Here's how the part is built. I have some questions about the finished solid (model axes, mm). Face numbers are marked on the shaded views. Give positions to 0.01 mm unless a question says otherwise; leave off trailing zeros. Order: outer loops, then holes, each group sorted by start corner. A loop starts at its lowest first (then second) coordinate and runs counter-clockwise, first axis right, second up. Notation, with made-up numbers: M 25.5,-27 L 32.5,-27 A16 cw 32.5,-20 Z; hole C -14.75,-24 d8. An arc over 180 degrees is marked long. Use CSV: the item, a comma, the result in double quotes. Start each with the question number.
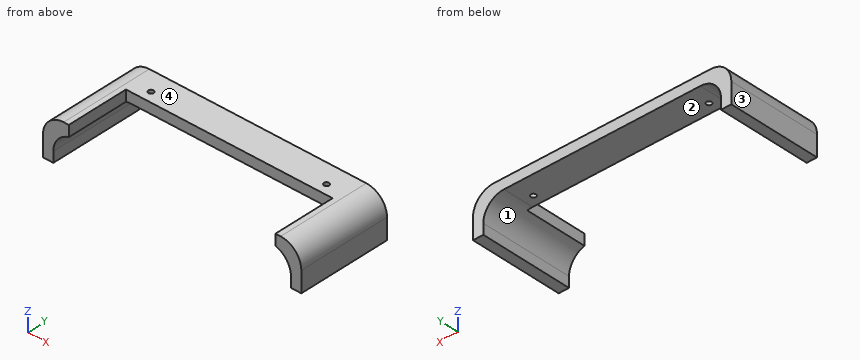
```python
from build123d import *

# Parameters (mm, degrees)
SKETCH1_W               = 250
SKETCH1_H               = 250
SKETCH1_W_2             = 230
SKETCH1_H_2             = 230
BOSS_EXTRUDE1_DEPTH     = 90
SKETCH2_W               = 200
SKETCH2_H               = 60
CUT_EXTRUDE1_DEPTH      = 50
FILLET1_R               = 20
SKETCH10_W              = 210
SKETCH10_H              = 90
CUT_EXTRUDE6_DEPTH      = 1
CUT_EXTRUDE6_DEPTH_BACK = 251
SKETCH11_R              = 2.5
CUT_EXTRUDE7_DEPTH      = 10


with BuildPart() as part:
    # Sketch1 → Boss-Extrude1 (new body)
    with BuildSketch(Plane(origin=(0, 0, 0), x_dir=(1, 0, 0), z_dir=(0, 1, 0))):
        Rectangle(SKETCH1_W, SKETCH1_H)
        Rectangle(SKETCH1_W_2, SKETCH1_H_2, mode=Mode.SUBTRACT)
    extrude(amount=BOSS_EXTRUDE1_DEPTH)

    # Sketch2 → Cut-Extrude1 (cut)
    with BuildSketch(Plane.XY.offset(125)):
        with Locations((0, 30)):
            Rectangle(SKETCH2_W, SKETCH2_H)
    extrude(amount=-CUT_EXTRUDE1_DEPTH, mode=Mode.SUBTRACT)

    # Fillet1
    fillet1_edges = [part.edges().sort_by_distance(p)[0] for p in [
        (-115, 45, 115),
        (115, 45, 115),
        (115, 45, -115),
        (-115, 45, -115),
        (-125, 45, 125),
        (125, 45, 125),
        (125, 45, -125),
        (-125, 45, -125),
    ]]
    fillet(fillet1_edges, radius=FILLET1_R)

    # Sketch10 → Cut-Extrude6 (cut, two sides)
    with BuildSketch(Plane(origin=(125, 0, 0), x_dir=(0, 0, -1), z_dir=(1, 0, 0))) as cut_extrude6_sk:
        with Locations((20, 45)):
            Rectangle(SKETCH10_W, SKETCH10_H)
    extrude(amount=CUT_EXTRUDE6_DEPTH, mode=Mode.SUBTRACT)
    extrude(cut_extrude6_sk.sketch, amount=-CUT_EXTRUDE6_DEPTH_BACK, mode=Mode.SUBTRACT)

    # Sketch11 → Cut-Extrude7 (cut)
    with BuildSketch(Plane.XY.offset(125)):
        with Locations((-85, 70)):
            Circle(SKETCH11_R)
        with Locations((85, 70)):
            Circle(SKETCH11_R)
    extrude(amount=-CUT_EXTRUDE7_DEPTH, mode=Mode.SUBTRACT)


solid = part.part
```
Q1. Imagine slicing it at A-A, the plane x = 85. Please give me the cut outline in (y, z).
Q2. Imagine slicing it at B-B, the plane z = 122.5. Please give me the cut outline in (x, y).
Q3. I need wall thicknesses on line 1 (Y direction, x = 85, z = 117.75); line 2 (Y direction, x = -66, z = 118); line 3 (Z direction, x = -96, y = 71.5). Which ranges of each line are inside material? Lowest first, please. Write a range as [from, to].
Q4. For P1, Ø5.5, axis at x = -41.5, z = 120.5, coming from the -Y side; P2, Ø8.5, axis at y = 22.5, z = 117, coming from the -X side; P3, Ø3, axis at x = 85, y = 70, coming from the -Z side; P4, Ø24, axis at x = -2.5, y = 73.5, coming from the -Z side, each with a flat end and sliding along its axis, tell me the tip position at first contact or that it passes through.
Q5. We'd pull the mould along X, two halves only. Please class the marked faces 1, 2, 3 and 4: pulls with the +X half, pulls with the -X half, needs draft (parallel to the pull), parting line crosses it, or undercut.
Q6. Imagine slicing it at D-D, the plane x = -40. Please give me the cut outline in (y, z).
Q7. Imagine slicing it at C-C, the plane y = 80.5. Please give me the cut outline in (x, z).
Reply:
1,outline,"M 60,115 L 67.5,115 L 67.5,125 L 60,125 Z; M 72.5,115 L 90,115 L 90,125 L 72.5,125 Z"
2,outline,"M -114.68,0 L -100,0 L -100,60 L 100,60 L 100,0 L 114.68,0 L 114.68,90 L -114.68,90 Z; hole C -85,70 d5; hole C 85,70 d5"
3,line 1,"y = [60, 67.5], [72.5, 90]"
3,line 2,"y = [60, 90]"
3,line 3,"z = [114.97, 125]"
4,P1,"stops at y = 60"
4,P2,"stops at x = -123.44"
4,P3,"passes through"
4,P4,"stops at z = 115"
5,face 1,"undercut"
5,face 2,"undercut"
5,face 3,"pulls with the -X half"
5,face 4,"needs draft"
6,outline,"M 60,115 L 90,115 L 90,125 L 60,125 Z"
7,outline,"M -125,85 L -115,85 L -115,95 A20 cw -95,115 L 95,115 A20 cw 115,95 L 115,85 L 125,85 L 125,105 A20 ccw 105,125 L -105,125 A20 ccw -125,105 Z"
